Autodesk Inventor part; units mm, degrees
ref_plane "Work Plane3" through (0, 0, -51) normal (0, 0, 1) x (1, 0, 0)
ref_plane "YZ Plane" through (0, 0, 0) normal (1, 0, 0) x (0, 1, 0)
ref_plane "XZ Plane" through (0, 0, 0) normal (0, 1, 0) x (-1, 0, 0)
sketch "Sketch1" plane through (0, 0, 0) normal (0, 0, 1) x (1, 0, 0)
  line L0 (79.3694, 29.7923) -> (84.3694, 29.7923)
  line L1 (84.3694, 29.7923) -> (84.3694, -15.2077)
  line L2 (84.3694, -15.2077) -> (-65.6306, -15.2077)
  line L3 (-65.6306, -15.2077) -> (-65.6306, -5.2077)
  line L4 (-65.6306, -5.2077) -> (79.3694, -5.2077)
  line L5 (79.3694, -5.2077) -> (79.3694, 29.7923)
  line L6 (79.3694, 29.7923) -> (84.3694, 29.7923)
  point P0 (0, 0)
  dimension "d0" = 45
  dimension "d1" = 150
  dimension "d2" = 10
  dimension "d3" = 5
extrude "Extrusion1" add sketch "Sketch1" against normal blind 82
fillet "Fillet1" radius 3 1 edges at (79.3694, 29.7923, -41)
fillet "Fillet2" radius 2 1 edges at (79.3694, -5.2077, -41)
ref_plane "Work Plane1" through (0, 0, -21) normal (0, 0, 1) x (1, 0, 0)
sketch "Sketch2" plane through (0, 0, -21) normal (0, 0, 1) x (1, 0, 0)
  point P0 (0, 0)
sketch "Sketch3" plane through (0, 0, -21) normal (0, 0, 1) x (1, 0, 0)
  line L0 (-65.6306, -15.2077) -> (-65.6306, -5.2077)
  line L1 (-65.6306, -5.2077) -> (-65.6306, 9.7923)
  line L2 (-65.6306, 9.7923) -> (42.3694, 28.5423)
  line L3 (-65.6306, -5.2077) -> (77.3694, -5.2077)
  line L4 (54.3694, -5.2077) -> (84.3564, -5.2077)
  arc A0 (77.3694, -5.2077) -> (79.3694, -3.2077) centre (77.3694, -3.2077) ccw
  line L5 (77.3694, -5.2077) -> (79.3694, -3.2077)
  line L6 (79.3694, -3.2077) -> (79.3694, 26.9279)
  line L7 (79.3694, 26.9279) -> (81.3477, 29.7923)
  line L8 (81.3477, 29.7923) -> (82.0785, 29.7923)
  line L9 (82.3694, 29.7923) -> (84.3694, 29.7923)
  line L10 (82.0785, 29.7923) -> (84.3694, 29.7923)
  line L11 (84.3694, 29.7923) -> (84.3694, 74.7923)
  line L12 (84.3694, 74.7923) -> (42.3694, 74.7923)
  line L13 (42.3694, 74.7923) -> (42.3694, 28.5423)
  point P0 (0, 0)
  point P1 (77.3694, -5.2077)
  dimension "d9" = 15
  dimension "d12" = 108
  dimension "d13" = 25
  dimension "d21" = 45
  dimension "d23" = 42
extrude "Extrusion2" add sketch "Sketch3" against normal blind 10 contours L1 L2 L13 L12 L11 L9 L10 L8 L7 L6 L5 L3
fillet "Fillet4" radius 21 2 edges at (84.3694, 74.7923, -26) (42.3694, 74.7923, -26)
fillet "Fillet5" radius 15 1 edges at (-65.6306, 9.7923, -26)
sketch "Sketch4" plane through (0, 0, -21) normal (0, 0, 1) x (1, 0, 0)
  point P0 (0, 0)
ref_plane "Work Plane3" through (0, 0, -51) normal (0, 0, 1) x (1, 0, 0)
sketch "Sketch6" plane through (0, 0, -51) normal (0, 0, 1) x (1, 0, 0)
  line L0 (77.3694, -5.2077) -> (-65.6306, -5.2077)
  arc A0 (-53.1963, 11.951) -> (-65.6306, -2.8279) centre (-50.6306, -2.8279) ccw
  line L1 (-65.6306, -2.8279) -> (-65.6306, -5.2077)
  line L2 (77.3694, -5.2077) -> (-65.6306, -5.2077)
  line L3 (77.3694, -5.2077) -> (79.3694, -3.2077)
  line L4 (79.3694, 26.7923) -> (79.3694, -3.2077)
  line L5 (79.3694, 26.7923) -> (79.3694, 26.9279)
  line L6 (79.3694, 26.9279) -> (79.3727, 26.9326)
  arc A1 (81.1769, 29.5451) -> (79.3727, 26.9326) centre (82.3694, 26.7923) ccw
  line L7 (81.1769, 29.5451) -> (81.3477, 29.7923)
  line L8 (81.3477, 29.7923) -> (82.3694, 29.7923)
  line L9 (84.3694, 29.7923) -> (82.3694, 29.7923)
  line L10 (84.3694, 29.7923) -> (84.3694, 53.7923)
  arc A2 (84.3694, 53.7923) -> (42.3694, 53.7923) centre (63.3694, 53.7923) ccw
  line L11 (42.3694, 53.7923) -> (42.3694, 28.5423)
  line L12 (42.3694, 28.5423) -> (-53.1963, 11.951)
  point P0 (0, 0)
extrude "Extrusion3" add sketch "Sketch6" against normal blind 10
sketch "Sketch7" plane through (0, 0, -21) normal (0, 0, 1) x (1, 0, 0)
  line L0 (-65.6306, -5.2077) -> (77.3694, -5.2077)
  line L1 (-65.6306, -5.2077) -> (77.3694, -5.2077)
  line L2 (-53.1963, 11.951) -> (42.3694, 28.5423)
  arc A0 (-53.1963, 11.951) -> (-65.6306, -2.8279) centre (-50.6306, -2.8279) ccw
  circle A1 centre (-50.6306, 2.2923) radius 3.75
  line L3 (42.3694, 53.7923) -> (42.3694, 28.5423)
  arc A2 (84.3694, 53.7923) -> (42.3694, 53.7923) centre (63.3694, 53.7923) ccw
  circle A3 centre (63.3694, 53.7923) radius 8
  point P0 (0, 0)
  point P1 (-50.6306, -5.2077)
  dimension "d29" = 15
  dimension "d30" = 7.5
  dimension "d31" = 7.5
  dimension "d34" = 16
extrude "Extrusion4" cut sketch "Sketch7" against normal blind 40 contours A1
sketch "Sketch8" plane through (0, 0, -21) normal (0, 0, 1) x (1, 0, 0)
  arc A0 (84.3694, 53.7923) -> (42.3694, 53.7923) centre (63.3694, 53.7923) ccw
  circle A1 centre (63.3694, 53.7923) radius 8
  point P0 (0, 0)
  dimension "d35" = 16
extrude "Extrusion5" cut sketch "Sketch8" against normal blind 40
fillet "Fillet6" radius 2 2 edges at (42.3694, 28.5423, -26) (42.3694, 28.5423, -56)
The listing builds one solid part. Answer for the finished solid, in the listing's coordinates (mm). A direction names the side the tool comes from. Give positions to 0.01 mm unless a question says otherwise; leave off trailing zeros. Loops run counter-clockwise (first coordinate to the right, second up) from the corner with the lowest first, then second, coordinate; pieces in that order, holes last. Notation, with made-up numbers: (48.5, 52.25) - (80.5, 52.25) arc R37 ccw to (80.5, 90.25) - close; hole circle Ø6 at (-8.5, -2). An arc over 180 degrees is marked (long way). Answer as a JSON object with one key per item and string values.
1. Flat-ended cylindrical pins translate along their axes: pin 1 Ø8 at (x, y) = (22.5, 24.5) entering from +Z; pin 2 Ø8 at (y, z) = (47, -24) entering from -X; pin 3 Ø6.5 at (y, z) = (17, -70.5) entering from -X; pin 4 Ø4.5 at (x, y) = (-50.63, 2.29) entering from +Z. Find the tip coordinate at first contact, or state that the pin passes through.
Determined:
{"pin 1": "z = -21", "pin 2": "x = 42.37", "pin 3": "x = 79.37", "pin 4": "through"}
2. A cutting plane is placed at C-C (z = -66). Write down the section's boundary in (x, y), then the cut area to 3 significant figures.
Determined:
{"outline": "(-65.63, -15.21) - (84.37, -15.21) - (84.37, 29.79) - (82.37, 29.79) arc R3 ccw to (79.37, 26.79) - (79.37, -3.21) arc R2 cw to (77.37, -5.21) - (-65.63, -5.21) - close", "area": "1,670 mm²"}
3. A cutting plane is placed at A-A (y = 57). Write down the section's boundary in (x, z), then the cut area to 3 significant figures.
Determined:
{"outline": "(42.62, -61) - (56.04, -61) - (56.04, -51) - (42.62, -51) - close; (42.62, -31) - (56.04, -31) - (56.04, -21) - (42.62, -21) - close; (70.7, -61) - (84.12, -61) - (84.12, -51) - (70.7, -51) - close; (70.7, -31) - (84.12, -31) - (84.12, -21) - (70.7, -21) - close", "area": "537 mm²"}
4. A cutting plane is placed at D-D (x = -23.5). Write down the section's boundary in (y, z).
Determined:
{"outline": "(-15.21, -82) - (-5.21, -82) - (-5.21, -61) - (17.11, -61) - (17.11, -51) - (-5.21, -51) - (-5.21, -31) - (17.11, -31) - (17.11, -21) - (-5.21, -21) - (-5.21, 0) - (-15.21, 0) - close"}
5. For faces 1 (the flat face through (79.369, 12, -71)), 2 (the flat face through (42.369, 42, -26)), 3 (the cylindrical face through (78.055, 68.804, -26.07)), 4 (the flat face through (5, -5.208, -41)), 5 (the flat face through (15, -9, 0)), determine the directions among +Z, -Z, +X, -X, +Y, -Y from which every point of the face is accessible in a straight line to the end or side of a thin tool.
Determined:
{"face 1": "-Z, -X, +Y", "face 2": "+Z, -Z, -X, +Y", "face 3": "+Z, -Z, +X, +Y", "face 4": "-X, +Y", "face 5": "+Z, +X, -X, +Y, -Y"}
6. For a pull along Z with two mould halves and no side action, classify faces 6 (the flat face through (79.369, 12, -10)), 7 (the flat face through (25, 18, -21)), 8 (the flat face through (79.369, 12, -41)) as pulls with the +Z half, pulls with the -Z half, needs draft (parallel to the pull), parting line crosses it, or undercut.
Determined:
{"face 6": "needs draft", "face 7": "pulls with the +Z half", "face 8": "undercut"}
7. Find the intervals of material crossed by L1, parallel to Z at x = 37, y = 25; L2, parallel to Y at x = 63, z = -41; L3, parallel to X at y = 45, z = -60, in increasing order. Write a range as [from, to].
Determined:
{"L1": "[-61, -51], [-31, -21]", "L2": "[-15.21, -5.21]", "L3": "[42.37, 84.37]"}
